```python
from build123d import *

# Parameters (mm, degrees)
F0_W     = 140
F0_H     = 200
F1_DEPTH = 25
F2_R     = 10
F3_T     = -4
F5_DEPTH = 2
F6_R     = 2.5
F7_DEPTH = 26
F8_R     = 2.5
F9_DEPTH = 6


with BuildPart() as f1:
    # F0 (on Top) → F1 (new body)
    with BuildSketch(Plane.XY):
        with Locations((-70, 100)):
            Rectangle(F0_W, F0_H)
    extrude(amount=F1_DEPTH)

    # F2
    f2_edges = [f1.edges().sort_by_distance(p)[0] for p in [
        (-70, 0, 0),
        (-140, 100, 0),
        (-70, 200, 0),
        (0, 100, 0),
        (-140, 0, 12.5),
        (0, 0, 12.5),
        (0, 200, 12.5),
        (-140, 200, 12.5),
    ]]
    fillet(f2_edges, radius=F2_R)

    # F3
    f3_openings = [f1.faces().sort_by_distance(p)[0] for p in [
        (-70, 100, 25),
    ]]
    offset(amount=F3_T, openings=f3_openings)

    # F4 (on face) → F5 (cut)
    with BuildSketch(Plane.XY.offset(25)):
        with BuildLine():
            Line((-2.5, 10), (-2.5, 190))
            ThreePointArc((-2.5, 190), (-4.6966991411, 195.3033008589), (-10, 197.5))
            Line((-10, 197.5), (-130, 197.5))
            ThreePointArc((-130, 197.5), (-135.3033008589, 195.3033008589), (-137.5, 190))
            Line((-137.5, 190), (-137.5, 10))
            ThreePointArc((-137.5, 10), (-135.3033008589, 4.6966991411), (-130, 2.5))
            Line((-130, 2.5), (-10, 2.5))
            ThreePointArc((-10, 2.5), (-4.6966991411, 4.6966991411), (-2.5, 10))
        make_face()
        with BuildLine():
            ThreePointArc((-136, 190), (-134.2426406871, 194.2426406871), (-130, 196))
            Line((-130, 196), (-10, 196))
            ThreePointArc((-10, 196), (-5.7573593129, 194.2426406871), (-4, 190))
            Line((-4, 190), (-4, 10))
            ThreePointArc((-4, 10), (-5.7573593129, 5.7573593129), (-10, 4))
            Line((-10, 4), (-130, 4))
            ThreePointArc((-130, 4), (-134.2426406871, 5.7573593129), (-136, 10))
            Line((-136, 10), (-136, 190))
        make_face(mode=Mode.SUBTRACT)
    extrude(amount=-F5_DEPTH, mode=Mode.SUBTRACT)

    # F6 (on face) → F7 (join)
    with BuildSketch(Plane.XY.offset(4)):
        with Locations((-127, 182.5)):
            Circle(F6_R)
        with Locations((-13, 182.5)):
            Circle(F6_R)
        with Locations((-127, 17.5)):
            Circle(F6_R)
        with Locations((-13, 17.5)):
            Circle(F6_R)
    extrude(amount=F7_DEPTH)

    # F8 (on face) → F9 (cut)
    with BuildSketch(Plane.XY.offset(30)):
        with Locations((-127, 182.5)):
            Circle(F8_R)
    extrude(amount=-F9_DEPTH, mode=Mode.SUBTRACT)


solid = f1.part
```
Work out the finished part from the listing and answer in its coordinate system (mm). A direction names the side the tool comes from. Round coordinates to 2 decimals unless told otherwise and drop trailing zeros. Loops run counter-clockwise (first coordinate to the right, second up) from the corner with the lowest first, then second, coordinate; pieces in that order, holes last. Notation, with made-up numbers: M 28,-6 L 52,-6 A26 ccw 52,18 Z; hole C 67,39 d6. An arc over 180 degrees is marked long. Use CSV: the item, a comma, the result in double quotes.
Q1. Each of these flat-tipped pins is pushed along its axis until it touches: pin 1 (3 mm diameter, centred on x = -101.5, y = 52, fed in from +Z); pin 2 (3 mm diameter, centred on x = -34, z = 8, fed in from +Y); pin 3 (5.5 mm diameter, centred on x = -126, y = 182, fed in from +Z). Where does it stop, or does it pass through?
Determined:
pin 1,"z = 4"
pin 2,"y = 199.99"
pin 3,"z = 24"
Q2. The mould has two halves that part along Y. Classify faces 1 (the cylindrical face through (-4.755, 4.639, 24.014)), 2 (the flat face through (-140, 99, 17)), 3 (the cylindrical face through (-137.15, 3.01, 17.6)): pulls with the +Y half, pulls with the -Y half, needs draft (parallel to the pull), parting line crosses it, or undercut.
Determined:
face 1,"undercut"
face 2,"needs draft"
face 3,"pulls with the -Y half"
Q3. Section B-B, the plane y = 182.5 is taken. Determine the outline of the cut face in (x, z), then the cut area to 3 significant figures.
Determined:
outline,"M -140,10 A10 ccw -130,0 L -10,0 A10 ccw 0,10 L 0,25 L -2.5,25 L -2.5,23 L -4,23 L -4,10 A6 cw -10,4 L -10.5,4 L -10.5,30 L -15.5,30 L -15.5,4 L -124.5,4 L -124.5,24 L -129.5,24 L -129.5,4 L -130,4 A6 cw -136,10 L -136,23 L -137.5,23 L -137.5,25 L -140,25 Z"
area,"925 mm2"
Q4. Section C-C, the plane x = -91.5 is taken. Determine the outline of the cut face in (y, z), then the cut area to 3 significant figures.
Determined:
outline,"M 0,10 A10 ccw 10,0 L 190,0 A10 ccw 200,10 L 200,25 L 197.5,25 L 197.5,23 L 196,23 L 196,10 A6 cw 190,4 L 10,4 A6 cw 4,10 L 4,23 L 2.5,23 L 2.5,25 L 0,25 Z"
area,"935 mm2"
Q5. A tool of negligible diameter and unlimited length cuts with its end or side. For faces 4 (the cylindrical face through (-2.85, 196.99, 17.6)), 5 (the cylindrical face through (-69.16, 5.711, 5.804)), from which of +Z, -Z, +X, -X, +Y, -Y can it reach the whole face along a straight path? Write none if from no direction.
Determined:
face 4,"+Z, -Z, +X, +Y"
face 5,"+Z"
Q6. Section A-A, the plane z = 19 is taken. Determine the outline of the cut face in (x, y).
Determined:
outline,"M -140,10 A10 ccw -130,0 L -10,0 A10 ccw 0,10 L 0,190 A10 ccw -10,200 L -130,200 A10 ccw -140,190 Z; C -127,17.5 d5; C -127,182.5 d5; C -13,17.5 d5; C -13,182.5 d5; hole M -136,10 A6 ccw -130,4 L -10,4 A6 ccw -4,10 L -4,190 A6 ccw -10,196 L -130,196 A6 ccw -136,190 Z"
Q7. Consider L1, parallel to X at y = 182.5, z = 21.25; L2, parallel to X at y = 88, z = 23.5; L3, parallel to X at y = 43, z = 19. Determine where each line is inside the solid, lowest interval first.
Determined:
L1,"-140 to -136, -129.5 to -124.5, -15.5 to -10.5, -4 to 0"
L2,"-140 to -137.5, -2.5 to 0"
L3,"-140 to -136, -4 to 0"
Q8. Section D-D, the plane z = 28 is taken. Determine the outline of the cut face in (x, y), then the cut area to 3 significant figures.
Determined:
outline,"C -127,17.5 d5; C -13,17.5 d5; C -13,182.5 d5"
area,"58.9 mm2"
